Here's how the part is built. I have some questions about the finished solid (model axes, mm). Coordinates: 2 decimals unless noted, no trailing zeros. Write each loop counter-clockwise with the first axis right and the second up, starting at its lowest first coordinate (ties: lowest second). Pieces come first, ordered by that corner, then holes. Notation, with made-up numbers: M 18,80.5 L 38,80.5 A20 cw 38,88.5 Z; hole C 89,21.25 d5. An arc over 180 degrees is marked long. Use a Markdown table: item, result.
```python
from build123d import *

# Parameters (mm, degrees)
SKETCH_1_R      = 0.8
EXTRUDE_1_DEPTH = 1


with BuildPart() as part:
    # Эскиз1 → Бобышка-Вытянуть1 (new body)
    with BuildSketch(Plane.XY):
        with BuildLine():
            Line((0, 40.912878475), (0, 43))
            ThreePointArc((0, 43), (-0.585786438, 44.414213562), (-2, 45))
            Line((-2, 45), (-45.727453461, 45))
            ThreePointArc((-45.727453461, 45), (-47.216544225, 44.335143699), (-47.715603611, 42.782608696))
            ThreePointArc((-47.715603611, 42.782608696), (-39.188772883, 20.282855848), (-20.814645128, 4.747826087))
            ThreePointArc((-20.814645128, 4.747826087), (-18.482786396, 5.188016153), (-18.212814487, 7.545652174))
            ThreePointArc((-18.212814487, 7.545652174), (-18.614079194, 27.721936832), (-1.826086957, 38.92045426))
            ThreePointArc((-1.826086957, 38.92045426), (-0.525580438, 39.561550625), (0, 40.912878475))
        make_face()
        with Locations((-19.947368247, 6.55)):
            Circle(SKETCH_1_R, mode=Mode.SUBTRACT)
        with Locations((-45.727453461, 43)):
            Circle(SKETCH_1_R, mode=Mode.SUBTRACT)
        with Locations((-2, 43)):
            Circle(SKETCH_1_R, mode=Mode.SUBTRACT)
    extrude(amount=EXTRUDE_1_DEPTH)


solid = part.part
```
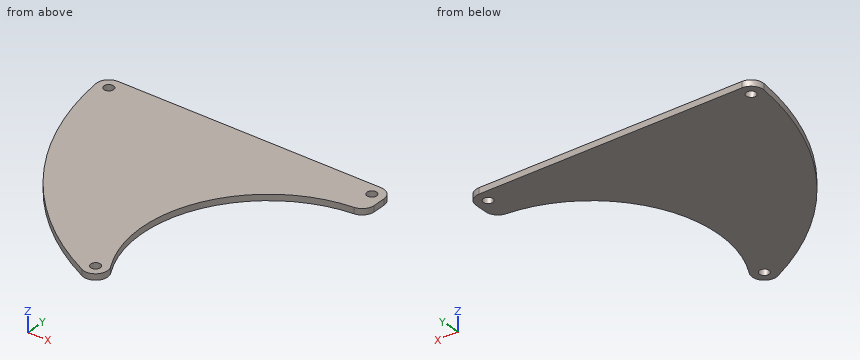
1. Will this pin go through, and if not, where does the flat tip stop? pin 1 Ø12 at (x, y) = (-7, 8.5) entering from +Z (1 decimal).
Answers follow:
| item | result |
|---|---|
| pin 1 | passes through |
2. I need wall thicknesses on probe 1 along X at (y, z) = (43, 0.2); probe 2 along Y at (x, z) = (-2.5, 0.45); probe 3 along X at (y, z) = (23, 0.6). Which ranges of each line are inside material? Lowest first, please.
Answers follow:
| item | result |
|---|---|
| probe 1 | x = -47.73 to -46.53, -44.93 to -2.8, -1.2 to 0 |
| probe 2 | y = 38.85 to 42.38, 43.62 to 45 |
| probe 3 | x = -40.98 to -20.4 |
3. Suppose I cut it at D-D on x = -7.5. Write out the boundary of the cut face in (y, z), and give its area (3 significant figures).
Answers follow:
| item | result |
|---|---|
| outline | M 37.62,0 L 45,0 L 45,1 L 37.62,1 Z |
| area | 7.38 mm2 |
4. Suppose I cut it at B-B on z = 0.25. Write out the boundary of the cut face in (x, y), and give its area (3 significant figures).
Answers follow:
| item | result |
|---|---|
| outline | M -47.72,42.78 A48 ccw -20.81,4.75 A2 ccw -18.21,7.55 A21 cw -1.83,38.92 A2 ccw 0,40.91 L 0,43 A2 ccw -2,45 L -45.73,45 A2 ccw Z; hole C -45.73,43 d1.6; hole C -19.95,6.55 d1.6; hole C -2,43 d1.6 |
| area | 983 mm2 |
5. Suppose I cut it at A-A on y = 6.55. Write out the boundary of the cut face in (x, z), and give its area (3 significant figures).
Answers follow:
| item | result |
|---|---|
| outline | M -24.21,0 L -20.75,0 L -20.75,1 L -24.21,1 Z; M -19.15,0 L -17.95,0 L -17.95,1 L -19.15,1 Z |
| area | 4.66 mm2 |
6. Suppose I cut it at C-C on y = 26. Write out the boundary of the cut face in (x, z).
Answers follow:
| item | result |
|---|---|
| outline | M -42.66,0 L -19.42,0 L -19.42,1 L -42.66,1 Z |
